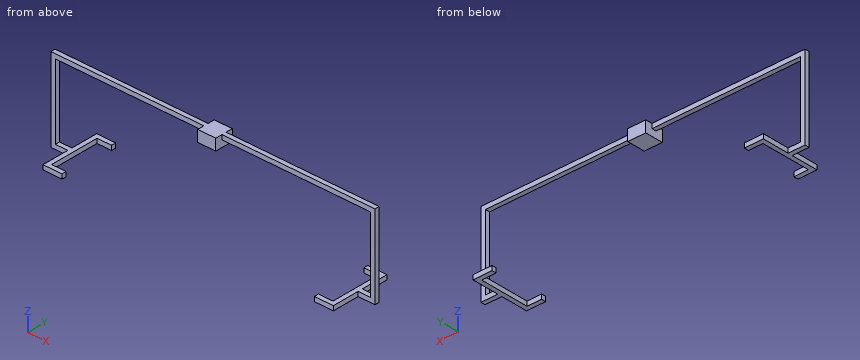
Autodesk Inventor part; units mm, degrees
ref_plane "Work Plane1" through (-720, 0, 0) normal (1, 0, 0) x (0, 0, -1)
ref_plane "YZ Plane" through (0, 0, 0) normal (1, 0, 0) x (0, 1, 0)
ref_plane "XZ Plane" through (0, 0, 0) normal (0, 1, 0) x (-1, 0, 0)
sketch "Sketch1" plane through (0, 0, 0) normal (0, 0, 1) x (1, 0, 0)
  line L0 (0, 0) -> (-1440, 0)
  line L1 (-1440, 0) -> (-1440, 20)
  line L2 (-1440, 20) -> (0, 20)
  line L3 (0, 20) -> (0, 0)
  dimension "d0" = 1440
  dimension "d1" = 20
extrude "Extrusion1" add sketch "Sketch1" along normal blind 20
sketch "Sketch2" plane through (0, 0, 20) normal (0, 0, 1) x (1, 0, 0)
  line L0 (-1440, 0) -> (0, 0)
  line L1 (0, 0) -> (0, 20)
  line L2 (0, 20) -> (-1440, 20)
  line L3 (-1440, 20) -> (-1440, 0)
  line L4 (0, 0) -> (-20, 0)
  line L5 (-20, 0) -> (-20, 20)
  line L6 (-20, 20) -> (0, 20)
  line L7 (0, 20) -> (0, 0)
  line L8 (-1440, 0) -> (-1420, 0)
  line L9 (-1420, 0) -> (-1420, 20)
  line L10 (-1420, 20) -> (-1440, 20)
  line L11 (-1440, 20) -> (-1440, 0)
  dimension "d4" = 20
  dimension "d5" = 20
extrude "Extrusion2" add sketch "Sketch2" along normal blind 350 contours L3 L2 L9 L0 | L5 L2 L1 L0
ref_plane "Work Plane1" through (-720, 0, 0) normal (1, 0, 0) x (0, 0, -1)
sketch "Sketch3" plane through (-720, 0, 0) normal (1, 0, 0) x (0, 0, -1)
  point P0 (0, 0)
sketch "Sketch4" plane through (-720, 0, 0) normal (1, 0, 0) x (0, 0, -1)
  line L0 (-20, 20) -> (-20, 0)
  line L1 (0, 0) -> (0, 20)
  line L2 (0, 0) -> (-370, 0)
  line L3 (-370, 20) -> (-370, 0)
  line L4 (0, 20) -> (-370, 20)
  line L5 (-20, 20) -> (0, 20)
  line L6 (0, 20) -> (0, 0)
  line L7 (0, 0) -> (-20, 0)
  line L8 (-20, 0) -> (-20, 20)
  point P0 (0, 0)
extrude "Extrusion3" cut sketch "Sketch4" along normal mid plane 1250 contours L4 L1 L2 L0
sketch "Sketch5" plane through (-1420, 0, 20) normal (1, 0, 0) x (0, 0, -1)
  line L0 (0, 20) -> (0, 0)
  line L1 (0, 20) -> (-350, 20)
  line L2 (-350, 0) -> (-350, 20)
  line L3 (0, 0) -> (-350, 0)
  line L4 (-350, 0) -> (-330, 0)
  line L5 (-330, 0) -> (-330, 20)
  line L6 (-330, 20) -> (-350, 20)
  line L7 (-350, 20) -> (-350, 0)
  point P0 (20, 0)
  dimension "d14" = 20
extrude "Extrusion4" add sketch "Sketch5" along normal blind 1401 contours L5 L3 L2 L1
sketch "Sketch7" plane through (-1440, 0, 370) normal (0, -1, 0) x (1, 0, 0)
  line L0 (95, -370) -> (95, -350)
  line L1 (20, -350) -> (95, -350)
  line L2 (20, -350) -> (20, -20)
  line L3 (20, -20) -> (1420, -20)
  line L4 (1420, -350) -> (1420, -20)
  line L5 (1345, -350) -> (1420, -350)
  line L6 (1345, -350) -> (1345, -370)
  line L7 (1440, -370) -> (1345, -370)
  line L8 (1440, -370) -> (1440, 0)
  line L9 (0, 0) -> (1440, 0)
  line L10 (0, -370) -> (0, 0)
  line L11 (95, -370) -> (0, -370)
  line L12 (1345, -370) -> (1365, -370)
  line L13 (1365, -370) -> (1365, -350)
  line L14 (1365, -350) -> (1345, -350)
  line L15 (1345, -350) -> (1345, -370)
  line L16 (20, -350) -> (95, -350)
  line L17 (95, -370) -> (75, -370)
  line L18 (75, -370) -> (75, -350)
  line L19 (75, -350) -> (95, -350)
  line L20 (95, -350) -> (95, -370)
  dimension "d23" = 20
  dimension "d24" = 20
extrude "Extrusion6" add sketch "Sketch7" along normal blind 120 contours L11 L18 L1 L0 | L7 L6 L5 L13
sketch "Sketch8" plane through (-1440, 20, 370) normal (0, 1, 0) x (1, 0, 0)
  line L0 (95, 350) -> (95, 370)
  line L1 (0, 370) -> (95, 370)
  line L2 (0, 370) -> (0, 0)
  line L3 (1440, 0) -> (0, 0)
  line L4 (1440, 370) -> (1440, 0)
  line L5 (1345, 370) -> (1440, 370)
  line L6 (1345, 370) -> (1345, 350)
  line L7 (1420, 350) -> (1345, 350)
  line L8 (1420, 350) -> (1420, 20)
  line L9 (20, 20) -> (1420, 20)
  line L10 (20, 350) -> (20, 20)
  line L11 (95, 350) -> (20, 350)
  line L12 (1345, 370) -> (1365, 370)
  line L13 (1365, 370) -> (1365, 350)
  line L14 (1365, 350) -> (1345, 350)
  line L15 (1345, 350) -> (1345, 370)
  line L16 (95, 370) -> (75, 370)
  line L17 (75, 370) -> (75, 350)
  line L18 (75, 350) -> (95, 350)
  line L19 (95, 350) -> (95, 370)
  dimension "d27" = 20
  dimension "d28" = 20
extrude "Extrusion7" add sketch "Sketch8" along normal blind 120 contours L11 L17 L1 L0 | L7 L6 L5 L13
sketch "Sketch9" plane through (-1345, 0, 0) normal (1, 0, 0) x (0, 0, -1)
  line L0 (-20, -120) -> (-20, 140)
  line L1 (0, -120) -> (-20, -120)
  line L2 (0, 140) -> (0, -120)
  line L3 (-20, 140) -> (0, 140)
  line L4 (-20, -120) -> (0, -120)
  line L5 (0, -120) -> (0, -100)
  line L6 (0, -100) -> (-20, -100)
  line L7 (-20, -100) -> (-20, -120)
  line L8 (0, 140) -> (0, -120)
  line L9 (-20, 140) -> (0, 140)
  line L10 (0, 140) -> (0, 120)
  line L11 (0, 120) -> (-20, 120)
  line L12 (-20, 120) -> (-20, 140)
  point P0 (0, 0)
  dimension "d35" = 20
  dimension "d36" = 20
extrude "Extrusion8" add sketch "Sketch9" along normal blind 1251 contours L0 L6 L2 L1 | L0 L3 L2 L11
sketch "Sketch10" plane through (-720, 0, 0) normal (1, 0, 0) x (0, 0, -1)
  line L0 (0, 0) -> (-20, 0)
  line L1 (0, 0) -> (0, -120)
  line L2 (-20, -120) -> (0, -120)
  line L3 (-20, 0) -> (-20, -120)
  line L4 (0, 120) -> (-20, 120)
  line L5 (0, 140) -> (-20, 140)
  line L6 (-20, 20) -> (-20, 140)
  line L7 (0, 20) -> (0, 140)
  line L8 (-20, -100) -> (0, -100)
  line L9 (-20, -120) -> (0, -120)
  line L10 (0, -120) -> (0, -100)
  line L11 (0, -100) -> (-20, -100)
  line L12 (-20, -100) -> (-20, -120)
  line L13 (-20, 120) -> (0, 120)
  line L14 (0, 120) -> (0, 140)
  line L15 (0, 140) -> (-20, 140)
  line L16 (-20, 140) -> (-20, 120)
  point P0 (0, 0)
extrude "Extrusion9" cut sketch "Sketch10" along normal mid plane 1120.8 contours L1 L2 L3 L8 | L4 L6 L5 L7
sketch "Sketch11" plane through (-720, 0, 0) normal (1, 0, 0) x (0, 0, -1)
  line L0 (-350, 20) -> (-350, 0)
  line L1 (-370, 20) -> (-370, 0)
  line L2 (0, 20) -> (-370, 20)
  line L3 (0, 0) -> (-370, 0)
  line L4 (-370, 50) -> (-320, 50)
  line L5 (-320, 50) -> (-320, -30)
  line L6 (-320, -30) -> (-370, -30)
  line L7 (-370, -30) -> (-370, 50)
  dimension "d49" = 50
  dimension "d50" = 80
  dimension "d51" = 30
extrude "Extrusion10" add sketch "Sketch11" along normal mid plane 80
properties part number "CameraMount"
Work out the finished part from the listing and answer in its coordinate system (mm). Give positions to 0.01 mm unless a question says otherwise; leave off trailing zeros. Order: outer loops, then holes, each group sorted by start corner. A loop starts at its lowest first (then second) coordinate and runs counter-clockwise, first axis right, second up. Notation, with made-up numbers: M 30,55.25 L 36,55.25 A21 cw 36,71.25 Z; hole C -22.75,60.25 d1. An arc over 180 degrees is marked long. Return JSON: item names as keys, results as strings.
Q1. Each of these flat-tipped pins is pushed along its axis until it touches: pin 1 (22 mm diameter, centred on x = -490.5, y = 14, fed in from -Z); pin 2 (6 mm diameter, centred on y = 58, z = 8, fed in from -X); pin 3 (10 mm diameter, centred on y = -43.5, z = 10.5, fed in from +X). Where does it stop, or does it pass through?
Answer below:
{"pin 1": "stops at z = 350", "pin 2": "stops at x = -1365", "pin 3": "stops at x = -75"}
Q2. Find section A-A, the plane z = 305. Write down the section's boundary in (x, y), and give its area (3 significant figures).
Answer below:
{"outline": "M -1440,0 L -1420,0 L -1420,20 L -1440,20 Z; M -20,0 L 0,0 L 0,20 L -20,20 Z", "area": "800 mm^2"}
Q3. Find the intervals of material crossed by line 1 along X through (y, z) = (-97, 15); line 2 along X through (y, z) = (14, 45); line 3 along Z through (x, y) = (-973.5, 3.5), in increasing order. Write a range as [from, to].
Answer below:
{"line 1": "x = [-1365, -1345], [-95, -75]", "line 2": "x = [-1440, -1420], [-20, 0]", "line 3": "z = [350, 370]"}
Q4. Find section B-B, the plane y = -63.5. Write down the section's boundary in (x, z), and give its area (3 significant figures).
Answer below:
{"outline": "M -1365,0 L -1345,0 L -1345,20 L -1365,20 Z; M -95,0 L -75,0 L -75,20 L -95,20 Z", "area": "800 mm^2"}
Q5. Find section C-C, the plane x = -369.5. Write down the section's boundary in (y, z).
Answer below:
{"outline": "M 0,350 L 20,350 L 20,370 L 0,370 Z"}
